Autodesk Inventor part; units mm, degrees
ref_plane "YZ Plane" through (0, 0, 0) normal (1, 0, 0) x (0, 1, 0)
ref_plane "XZ Plane" through (0, 0, 0) normal (0, 1, 0) x (-1, 0, 0)
ref_plane "XY Plane" through (0, 0, 0) normal (0, 0, 1) x (1, 0, 0)
sketch "Sketch1" plane through (0, 0, 0) normal (0, 1, 0) x (-1, 0, 0)
  line L0 (-11.4129, 10) -> (10.3431, 10)
  line L1 (20, 2) -> (20, -2)
  line L2 (10.3431, -10) -> (-17.4129, -10)
  line L3 (-20, -10) -> (-20, 10)
  line L4 (20, -10) -> (-20, 10) construction
  line L5 (20, 10) -> (-20, -10) construction
  line L6 (13.1716, -8.8284) -> (17.6284, -4.3716)
  line L7 (13.1716, 8.8284) -> (17.6284, 4.3716)
  line L8 (18.8, 1.5431) -> (18.8, -1.5431)
  arc A0 (18.8, 1.5431) -> (17.6284, 4.3716) centre (14.8, 1.5431) ccw
  arc A1 (17.6284, -4.3716) -> (18.8, -1.5431) centre (14.8, -1.5431) ccw
  arc A2 (13.1716, 8.8284) -> (10.3431, 10) centre (10.3431, 6) ccw
  arc A3 (10.3431, -10) -> (13.1716, -8.8284) centre (10.3431, -6) ccw
  line L9 (-18, -10) -> (-12, 10)
  line L10 (-12.5623, 10.1687) -> (-26.3566, 14.307)
  line L11 (-33.8781, 16.5634) -> (-39.8781, -3.4366)
  line L12 (-35.8836, -4.6349) -> (-18.5623, -9.8313)
  line L13 (-26.8781, 14.4634) -> (-37.0046, -4.2986)
  line L14 (-27.3388, 14.7536) -> (-59.1142, 34.7654)
  line L15 (-37.7675, -3.4111) -> (-65.2661, 28.5779)
  arc A4 (-12.5623, 10.1687) -> (-11.4129, 10) centre (-11.4129, 14) ccw
  arc A5 (-18.5623, -9.8313) -> (-17.4129, -10) centre (-17.4129, -6) ccw
  arc A6 (-27.3388, 14.7536) -> (-26.3566, 14.307) centre (-25.2072, 18.1383) ccw
  arc A7 (-37.7675, -3.4111) -> (-35.8836, -4.6349) centre (-34.7342, -0.8036) ccw
  arc A8 (-59.1142, 34.7654) -> (-65.2661, 28.5779) centre (-61.5814, 31.0663) ccw
  line L16 (18.8, 0) -> (8.8, 0)
  circle A9 centre (0.8, 0) radius 1.025
  circle A10 centre (8.8, -8) radius 1.025
  circle A11 centre (16.8, 0) radius 1.025
  circle A12 centre (8.8, 8) radius 1.025
  line L17 (-23.0219, -4.861) -> (-29.7868, -2.8316)
  line L18 (-22.3993, -4.5258) -> (-18.4228, 8.7292)
  line L19 (-19.263, 9.2186) -> (-30.0044, -2.007)
  arc A13 (-23.0219, -4.861) -> (-22.3993, -4.5258) centre (-22.8782, -4.3821) ccw
  arc A14 (-30.0044, -2.007) -> (-29.7868, -2.8316) centre (-29.6432, -2.3526) ccw
  arc A15 (-18.4228, 8.7292) -> (-19.263, 9.2186) centre (-18.9017, 8.8729) ccw
  line L20 (-37.6066, 5.1132) -> (-33.634, 12.4734)
  line L21 (-33.634, 12.4734) -> (-55.2323, 26.0758)
  line L22 (-55.8779, 25.3268) -> (-38.4257, 5.0247)
  arc A16 (-38.4257, 5.0247) -> (-37.6066, 5.1132) centre (-38.0466, 5.3506) ccw
  arc A17 (-55.2323, 26.0758) -> (-55.8779, 25.3268) centre (-55.4988, 25.6528) ccw
  point P0 (0, 0)
  point P1 (0, 0)
  point P2 (12, -10)
  point P3 (12, 10)
  point P4 (20, 10)
  point P5 (18.8, 3.2)
  point P6 (18.8, -3.2)
  point P7 (-37.9518, 4.4734)
  point P8 (-35.6203, 8.7933)
  dimension "d0" = 40
  dimension "d1" = 20
  dimension "d32" = 8
  dimension "d33" = 8
  dimension "d34" = 8
  dimension "d35" = 8
  dimension "d43" = 1.2
  dimension "d46" = 4
  dimension "d47" = 2
  dimension "d48" = 8
  dimension "d49" = 3
  dimension "d50" = 7
  dimension "d51" = 43.3541
  dimension "d52" = 32.617
  dimension "d53" = 4
  dimension "d54" = 10
  dimension "d55" = 2.05
  dimension "d56" = 8
  dimension "d59" = 360
  dimension "d79" = 0.5
  dimension "d80" = 8
  dimension "d81" = 5
  dimension "d82" = 5
  dimension "d83" = 0.5
extrude "Extrusion1" add sketch "Sketch1" along normal blind 3
sketch "Sketch8" plane through (0, 0, 0) normal (0, -1, 0) x (1, 0, 0)
  arc A0 (17.4129, -10) -> (18.5623, -9.8313) centre (17.4129, -6) ccw
  line L0 (-13.1716, -8.8284) -> (-17.6284, -4.3716)
  arc A1 (35.8836, -4.6349) -> (37.7675, -3.4111) centre (34.7342, -0.8036) ccw
  circle A2 centre (34.7342, -0.8036) radius 1.5
  circle A3 centre (30.2342, 11.6964) radius 1.5
  line L1 (65.2661, 28.5779) -> (37.7675, -3.4111)
  line L2 (27.3388, 14.7536) -> (59.1142, 34.7654)
  line L3 (15.9075, -6.542) -> (11.4075, 5.958)
  line L4 (14.4183, 7.042) -> (18.9183, -5.458)
  arc A4 (15.9075, -6.542) -> (18.9183, -5.458) centre (17.4129, -6) ccw
  arc A5 (14.4183, 7.042) -> (11.4075, 5.958) centre (12.9129, 6.5) ccw
  line L5 (34.7342, -0.8036) -> (30.2342, 11.6964) construction
  line L6 (36.1456, -0.2955) -> (31.6456, 12.2045)
  line L7 (28.8229, 11.1883) -> (33.3229, -1.3117)
  arc A6 (33.3229, -1.3117) -> (36.1456, -0.2955) centre (34.7342, -0.8036) ccw
  arc A7 (31.6456, 12.2045) -> (28.8229, 11.1883) centre (30.2342, 11.6964) ccw
  line L8 (59.3782, 24.0575) -> (55.8591, 30.2331) construction
  line L9 (60.5121, 24.7036) -> (56.993, 30.8792)
  line L10 (54.7253, 29.587) -> (58.2444, 23.4114)
  arc A8 (58.2444, 23.4114) -> (60.5121, 24.7036) centre (59.3782, 24.0575) ccw
  arc A9 (56.993, 30.8792) -> (54.7253, 29.587) centre (55.8591, 30.2331) ccw
  point P0 (0, 0)
  point P1 (17.9938, -9.9576)
  point P2 (15.1629, 0.25)
  point P3 (32.4842, 5.4464)
  point P4 (57.6187, 27.1453)
  dimension "d64" = 3
  dimension "d69" = 3
  dimension "d70" = 4.5
  dimension "d71" = 12.5
  dimension "d88" = 1.6
extrude "Extrusion7" add sketch "Sketch8" along normal blind 40
extrude "Extrusion8" add sketch "Sketch1" against normal blind 3 from surface at -40 contours A11 L16 | L16 A11 | L0 A2 L7 A0 L8 A1 L6 A3 L2 A5 L12 A7 L15 A8 L14 A6 L10 A4 | A9 | A10 | A12
sketch "Sketch10" plane through (-10.3431, -43, -10) normal (0, -1, 0) x (1, 0, 0)
  line L0 (-8.4569, 8.4569) -> (-8.4569, 11.5431)
  line L1 (-8.4569, 10) -> (1.5431, 10)
  circle A0 centre (1.5431, 10) radius 1.25
  point P0 (10.3431, 10)
  dimension "d84" = 10
  dimension "d85" = 2.5
extrude "Extrusion9" cut sketch "Sketch10" against normal blind 3
properties part number "leg_part"
Work out the finished part from the listing and answer in its coordinate system (mm). A direction names the side the tool comes from. Coordinates: 2 decimals unless noted, no trailing zeros. Order: outer loops, then holes, each group sorted by start corner. A loop starts at its lowest first (then second) coordinate and runs counter-clockwise, first axis right, second up. Notation, with made-up numbers: (51.5, 46) - (62.5, 46) arc R23 cw to (62.5, 69) - close; hole circle Ø8 at (79.5, 3). An arc over 180 degrees is marked (long way). Answer as a JSON object with one key per item and string values.
1. Consider line 1 (Z direction, x = -8.8, y = 1.1) (3 decimals); line 2 (Y direction, x = 16, z = 7); line 3 (X direction, y = -7, z = -1.5). Determine where each line is inside the solid, lowest interval first.
Output values:
{"line 1": "z = -10 to -9.025, -6.975 to 6.975, 9.025 to 10", "line 2": "y = -43 to -40, 0 to 3", "line 3": "x = 14.09 to 17.49, 33.41 to 36.06"}
2. Find section A-A on x = -0.8. Determine the outline of the cut face in (y, z) (3 decimals), plus the area to 3 significant figures.
Output values:
{"outline": "(-43, -10) - (-40, -10) - (-40, 10) - (-43, 10) - close; (0, -10) - (3, -10) - (3, -1.025) - (0, -1.025) - close; (0, 1.025) - (3, 1.025) - (3, 10) - (0, 10) - close", "area": "114 mm²"}
3. Each of these flat-tipped pins is pushed along its axis until it touches: P1, Ø4, axis at y = -5.5, z = 26, coming from the -X side; P2, Ø4, axis at y = -37, z = 21.5, coming from the +X side; P3, Ø12, axis at x = 19, y = -24, coming from the +Z side. Where does it stop, or does it pass through?
Output values:
{"P1": "stops at x = 55.63", "P2": "stops at x = 60.56", "P3": "stops at z = 8.1"}
4. Find section B-B on y = -39. Determine the outline of the cut face in (x, z).
Output values:
{"outline": "(11.41, 5.96) - (15.91, -6.54) arc R1.6 ccw to (18.92, -5.46) - (14.42, 7.04) arc R1.6 ccw to start; (28.82, 11.19) - (33.32, -1.31) arc R1.5 ccw to (36.15, -0.3) - (31.65, 12.2) arc R1.5 ccw to start; (54.73, 29.59) - (58.24, 23.41) arc R1.31 ccw to (60.51, 24.7) - (56.99, 30.88) arc R1.31 ccw to start"}
5. Find section D-D on x = 50. Determine the outline of the cut face in (y, z), plus the area to 3 significant figures.
Output values:
{"outline": "(-43, 10.82) - (-40, 10.82) - (-40, 18.49) - (-43, 18.49) - close; (-43, 22.78) - (-40, 22.78) - (-40, 29.03) - (-43, 29.03) - close; (0, 10.82) - (3, 10.82) - (3, 18.49) - (0, 18.49) - close; (0, 22.78) - (3, 22.78) - (3, 29.03) - (0, 29.03) - close", "area": "83.5 mm²"}
6. The mould has two halves that part along Z. Classify faces 3 (the face through (26.36, -41.48, -3.86)), 4 (the face through (36.927, -41.479, -4.149)), 5 (the face through (-18.504, -41.479, 3.054)), 6 (the face through (-9.778, 1.479, -8.308)): +Z half, -Z half, draft (parallel to the pull), parting line (faces both ways), or undercut.
Output values:
{"face 3": "undercut", "face 4": "-Z half", "face 5": "+Z half", "face 6": "undercut"}
7. A tool of negligible diameter and unlimited length cuts with its end or side. For faces 1 (the face through (13.69, -19.72, -0.38)), 2 (the face through (36.9, 1.479, -4.167)), from which of +Z, -Z, +X, -X, +Y, -Y can it reach the whole face along a straight path? Write none if from no direction.
Output values:
{"face 1": "-Z, -X", "face 2": "-Z, +X, +Y, -Y"}
8. Find section C-C on z = 17. Determine the outline of the cut face in (x, y).
Output values:
{"outline": "(30.91, -43) - (40.82, -43) - (40.82, -40) - (30.91, -40) - close; (30.91, 0) - (40.82, 0) - (40.82, 3) - (30.91, 3) - close; (48.72, -43) - (55.31, -43) - (55.31, -40) - (48.72, -40) - close; (48.72, 0) - (55.31, 0) - (55.31, 3) - (48.72, 3) - close"}
